Geometry check sheet. Reference: drawing and pictorial views, mm from the part's lowest x, y, z. Coordinates: 2 decimals unless noted, no trailing zeros. Loops run counter-clockwise (first coordinate to the right, second up) from the corner with the lowest first, then second, coordinate; pieces in that order, holes last. Notation, with made-up numbers: (-19.75, 26) -> (25.25, 26) arc R27 cw to (25.25, 44) -> close; hole circle Ø7 at (7, 13.5). An arc over 180 degrees is marked (long way). Answer as a JSON object with one key per item and string values. Group by question number.
Q1. Cross-section at B-B on y = 2. Record the boundary of the cut face in (x, z), and give its area (3 significant figures).
Q2. Cross-section at A-A on z = 75. Record the boundary of the cut face in (x, y).
Q3. Scan lines: L1, parallel to X at y = 1.5, z = 66.45; L2, parallel to Z at x = 12, y = 2.5; L3, parallel to X at y = 1.5, z = 90.05. Record each from-to range of solid material in increasing order.
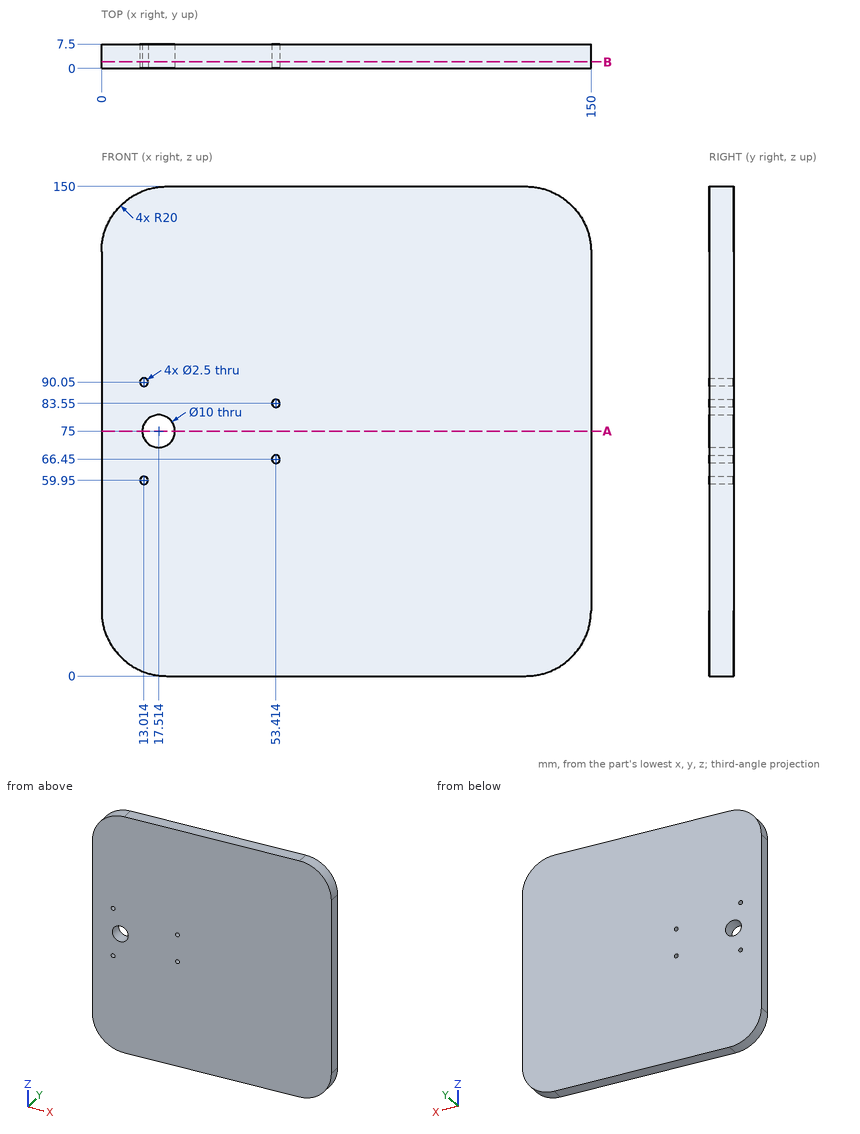
Computed values:
{
 "1": {"outline": "(0, 20) arc R20 ccw to (20, 0) -> (130, 0) arc R20 ccw to (150, 20) -> (150, 130) arc R20 ccw to (130, 150) -> (20, 150) arc R20 ccw to (0, 130) -> close; hole circle Ø2.5 at (13.01, 59.95); hole circle Ø2.5 at (13.01, 90.05); hole circle Ø10 at (17.51, 75); hole circle Ø2.5 at (53.41, 66.45); hole circle Ø2.5 at (53.41, 83.55)", "area": "22,100 mm²"},
 "2": {"outline": "(0, 0) -> (12.51, 0) -> (12.51, 7.5) -> (0, 7.5) -> close; (22.51, 0) -> (150, 0) -> (150, 7.5) -> (22.51, 7.5) -> close"},
 "3": {"L1": "x = 0 to 52.16, 54.66 to 150", "L2": "z = 1.67 to 59.22, 60.68 to 89.32, 90.78 to 148.33", "L3": "x = 0 to 11.76, 14.26 to 150"}
}
